Could you check a few things on this drawing? It's one solid part, dimensions in mm from its lowest x, y, z. A direction names the side the tool comes from. Round coordinates to 2 decimals unless told otherwise and drop trailing zeros. Write each loop counter-clockwise with the first axis right and the second up, starting at its lowest first coordinate (ties: lowest second). Pieces come first, ordered by that corner, then holes. Notation, with made-up numbers: (82, 9.5) -> (130, 9.5) arc R12 cw to (130, 17.5) -> close; hole circle Ø7 at (83, 32). An arc over 180 degrees is marked (long way). Answer in a Markdown table with one row per item. Add a question column.
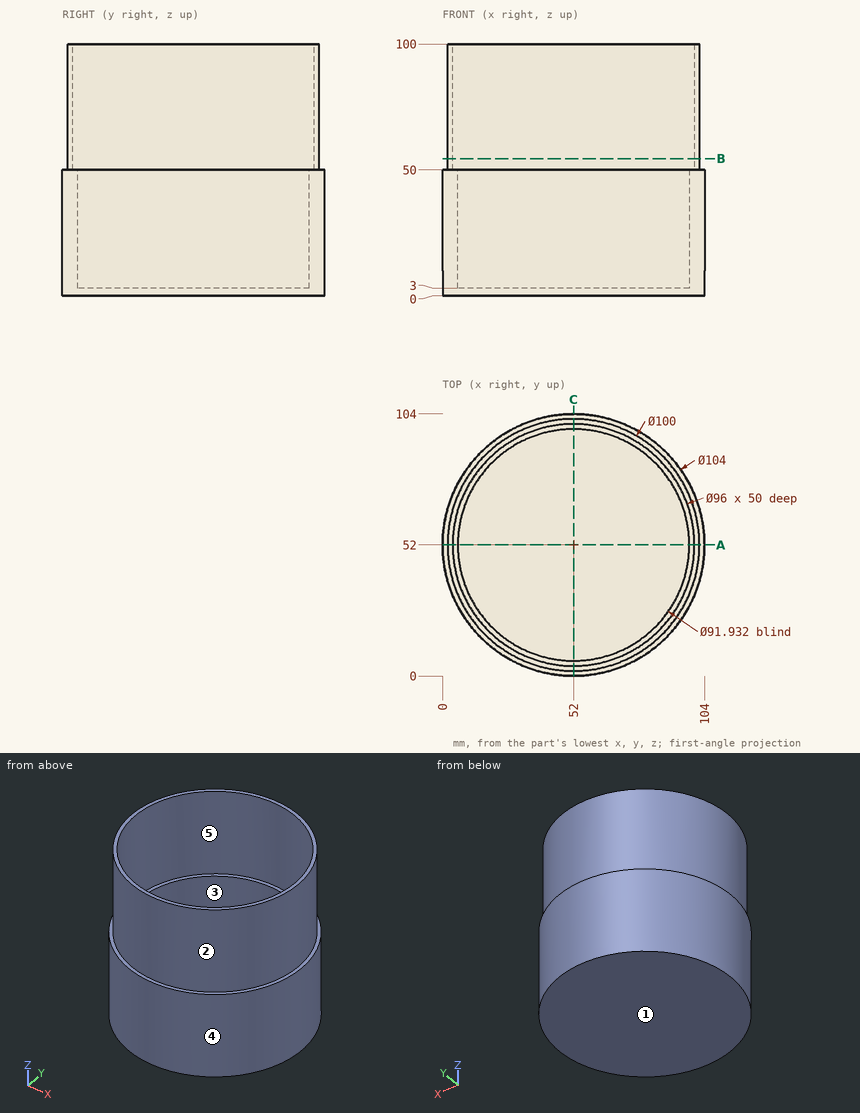
(1) If we mould it in two halves opening along Y, with no side actions, what happens to the marked faces 1, 2 and 3? For each: pulls with the +Y half, pulls with the -Y half, needs draft (parallel to the pull), parting line crosses it, or undercut.
(2) Suppose I cut it at A-A, the plane y = 52. Please give me the cut outline in (x, z).
(3) I need wall thicknesses on L1, parallel to Y at x = 52, z = 65; L2, parallel to Y at x = 52, z = 32.5; L3, parallel to Z at x = 38.5, y = 32. Which ranges of each line are inside material? Lowest first, please.
(4) For P1, Ø1, axis at y = 86, z = 24.5, coming from the -X side; P2, Ø5, axis at x = 66.5, z = 19.5, coming from the +Y side; P3, Ø3, axis at x = 32, z = 89.5, coming from the +Y side, each with a flat end and sliding along its axis, tell me the tip position at first contact or that it passes through.
(5) On a 3-axis mill with a long thin cutter (end or side, diameter ignored), from which of +Z, -Z, +X, -X, +Y, -Y can I reach the whole of each face in a straight line? I mean the marked faces 4 and 5. Say none if no direction works.
(6) Suppose I cut it at B-B, the plane z = 54.5. Please give me the cut outline in (x, y).
Response:
| question | item | result |
|---|---|---|
| 1 | face 1 | needs draft |
| 1 | face 2 | parting line crosses it |
| 1 | face 3 | undercut |
| 2 | outline | (0, 0) -> (104, 0) -> (104, 50) -> (102, 50) -> (102, 100) -> (100, 100) -> (100, 50) -> (97.97, 50) -> (97.97, 3) -> (6.03, 3) -> (6.03, 50) -> (4, 50) -> (4, 100) -> (2, 100) -> (2, 50) -> (0, 50) -> close |
| 3 | L1 | 2 to 4, 100 to 102 |
| 3 | L2 | 0 to 6.03, 97.97 to 104 |
| 3 | L3 | 0 to 3 |
| 4 | P1 | x = 12.23 |
| 4 | P2 | y = 102.6 |
| 4 | P3 | y = 98.45 |
| 5 | face 4 | +Z, -Z |
| 5 | face 5 | +Z |
| 6 | outline | circle Ø100 at (52, 52); hole circle Ø96 at (52, 52) |
